Build history of the part. All positions in model axes, mm. A direction names the side the tool comes from. Round coordinates to 2 decimals unless told otherwise and drop trailing zeros. Write each loop counter-clockwise with the first axis right and the second up, starting at its lowest first coordinate (ties: lowest second). Pieces come first, ordered by that corner, then holes. Notation, with made-up numbers: (82, 8.5) -> (90, 8.5) arc R19 cw to (90, 31.5) -> close; hole circle Ø10 at (69.25, 74.25). An arc over 180 degrees is marked (long way). Return JSON: item names as keys, results as strings.
from build123d import *

# Parameters (mm, degrees)
SKETCH2_R   = 3.175
SKETCH2_R_2 = 2.4638


with BuildPart() as part:
    # Sweep-Thin1: sweep along a path in Sketch1
    with BuildLine(Plane(origin=(0, 0, 0), x_dir=(1, 0, 0), z_dir=(0, 1, 0))) as sweep_thin1_path:
        Line((0, 0), (0, 14))
        ThreePointArc((0, 14), (4.686291501, 25.313708499), (16, 30))
        Line((16, 30), (17.2, 30))
        Line((17.2, 30), (30, 30))
    # Sketch2 → Sweep-Thin1 (sweep)
    with BuildSketch(Plane.XY):
        Circle(SKETCH2_R)
        Circle(SKETCH2_R_2, mode=Mode.SUBTRACT)
    sweep(path=sweep_thin1_path.line)


solid = part.part
Q1. Pin check, flat tips, straight feed: pin 1 Ø3 at (x, y) = (21.5, -2.5) entering from +Z; pin 2 Ø2 at (x, y) = (16.5, 0.5) entering from +Z; pin 3 Ø2 at (y, z) = (2.5, -20) entering from +X. Stop position of each tip, or through.
Verdict:
{"pin 1": "stops at z = -26.99", "pin 2": "stops at z = -26.82", "pin 3": "stops at x = 4.43"}
Q2. Saw through at A-A on y = 0. List the corners of the cut face in (x, z) (3 decimals).
Verdict:
{"outline": "(-3.175, -14) arc R19.175 ccw to (16, -33.175) -> (30, -33.175) -> (30, -32.464) -> (16, -32.464) arc R18.464 cw to (-2.464, -14) -> (-2.464, 0) -> (-3.175, 0) -> close; (2.464, -14) arc R13.536 ccw to (16, -27.536) -> (30, -27.536) -> (30, -26.825) -> (16, -26.825) arc R12.825 cw to (3.175, -14) -> (3.175, 0) -> (2.464, 0) -> close"}
Q3. Two-plate mould, pull along Y, no slides. Class faces 1 (the cylindrical face through (-0.69, 3.1, -7.1)), 2 (the flat face through (30, 2, -32)), 3 (the cylindrical face through (-2.46, -0.11, -7.1)): +Y half, -Y half, draft (parallel to the pull), parting line (faces both ways), or undercut.
Verdict:
{"face 1": "parting line", "face 2": "draft", "face 3": "undercut"}
Q4. 3-axis set-ups, long thin cutter, end or side, ignore diameter. For faces 4 (the cylindrical face through (23.1, -0.74, -27.65)), 5 (the flat face through (2, -2, 0)): which of +Z, -Z, +X, -X, +Y, -Y reach the whole face in a straight line?
Verdict:
{"face 4": "+X", "face 5": "+Z, +X, -X, +Y, -Y"}
Q5. Wall check: L1, parallel to Z at x = 22.25, y = 0 (3 decimals); L2, parallel to Y at x = 0, z = -3 (3 decimals); L3, parallel to X at y = 1, z = -18. Give the ranges that are in metal, low to high.
Verdict:
{"L1": "z = -33.175 to -32.464, -27.536 to -26.825", "L2": "y = -3.175 to -2.464, 2.464 to 3.175", "L3": "x = -2.59 to -1.81, 2.85 to 3.64"}
Q6. Saw through at B-B on x = 22. List the corners of the cut face in (y, z) (3 decimals), then the cut area to 3 significant figures.
Verdict:
{"outline": "circle Ø6.35 at (0, -30); hole circle Ø4.928 at (0, -30)", "area": "12.6 mm²"}
